Source: three-view drawing plus pictorial views. Frame: mm from the lowest corner of the part. A direction names the side the tool comes from. Round coordinates to 2 decimals unless told otherwise and drop trailing zeros. Loops run counter-clockwise (first coordinate to the right, second up) from the corner with the lowest first, then second, coordinate; pieces in that order, holes last. Notation, with made-up numbers: M -3.5,3.5 L 36.5,3.5 A11 ccw 36.5,15.5 Z; hole C 8.5,85 d1. An arc over 180 degrees is marked long. Return JSON: item names as keys, results as strings. Group by question number.
1) Section D-D (x = 22.25). Output: boundary loops of the cut face in (y, z).
2) Access query for the marked faces 1, 2 and 3. Directions: +Z, -Z, +X, -X, +Y, -Y. A direction counts if a zero-diameter tool reaches every point of the face in a straight line with its end or side. Return the directions, or none.
3) Contact query for flat-ended pins moving along their axis: P1, Ø2.5, axis at x = 12.5, y = 2.5, coming from the +Z side; P2, Ø12, axis at x = 14.5, y = 25.5, coming from the -Z side; P3, Ø8, axis at y = 26.5, z = 12.5, coming from the -X side; P4, Ø1.5, axis at x = 16, z = 1.5, coming from the +Y side. Output: stop coordinate, or through.
4) Section B-B (z = 7). Output: boundary loops of the cut face in (x, y).
5) Section A-A (x = 3.75). Output: boundary loops of the cut face in (y, z).
6) Material intervals for line 1 (X direction, y = 15, z = 10.25); line 2 (Y direction, x = 4.25, z = 10), sorted ascending. Write a range as from..to.
7) Section C-C (y = 7). Output: boundary loops of the cut face in (x, z).
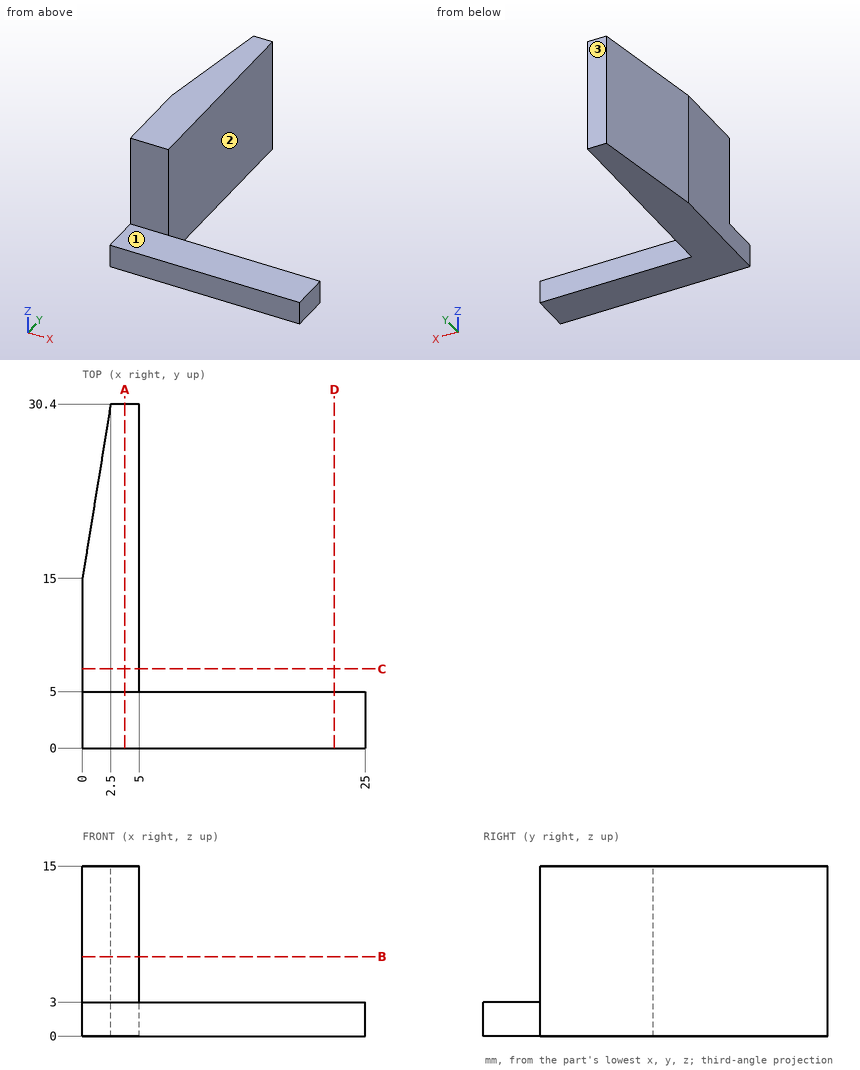
Returned:
{
 "1": {"outline": "M 0,0 L 5,0 L 5,3 L 0,3 Z"},
 "2": {"face 1": "+Z, +X, -X, -Y", "face 2": "+Z, -Z, +X, +Y", "face 3": "+Z, -Z, +X, -X, +Y"},
 "3": {"P1": "stops at z = 3", "P2": "passes through", "P3": "stops at x = 1.22", "P4": "stops at y = 5"},
 "4": {"outline": "M 0,5 L 5,5 L 5,30.4 L 2.5,30.4 L 0,15 Z"},
 "5": {"outline": "M 0,0 L 30.4,0 L 30.4,15 L 5,15 L 5,3 L 0,3 Z"},
 "6": {"line 1": "x = 0..5", "line 2": "y = 5..30.4"},
 "7": {"outline": "M 0,0 L 5,0 L 5,15 L 0,15 Z"}
}
